Work out the finished part from the listing and answer in its coordinate system (mm). A direction names the side the tool comes from. Give positions to 0.01 mm unless a question says otherwise; leave off trailing zeros. Order: outer loops, then holes, each group sorted by start corner. A loop starts at its lowest first (then second) coordinate and runs counter-clockwise, first axis right, second up. Notation, with made-up numbers: (81.5, -37) - (138.5, -37) arc R22 cw to (138.5, -5) - close; hole circle Ø11 at (-15, 11). An arc over 180 degrees is marked (long way). Put each result on its own line as item: value.
```python
from build123d import *

# Parameters (mm, degrees)
SKETCH1_R           = 5
SKETCH1_R_2         = 6
SKETCH1_R_3         = 30
BOSS_EXTRUDE1_DEPTH = 6


with BuildPart() as part:
    # Sketch1 → Boss-Extrude1 (new body)
    with BuildSketch(Plane.XY):
        with BuildLine():
            Line((-183.863104209, -89.445070531), (-97.598804033, -2.338194347))
            ThreePointArc((-97.598804033, -2.338194347), (-66.500702639, 38.39419857), (-46.774466313, 85.692140845))
            Line((-46.774466313, 85.692140845), (-14.469848781, 203.952654329))
            ThreePointArc((-14.469848781, 203.952654329), (0, 215), (14.469848781, 203.952654329))
            Line((14.469848781, 203.952654329), (46.774466313, 85.692140845))
            ThreePointArc((46.774466313, 85.692140845), (66.500702639, 38.39419857), (97.598804033, -2.338194347))
            Line((97.598804033, -2.338194347), (183.863104209, -89.445070531))
            ThreePointArc((183.863104209, -89.445070531), (186.195461814, -107.5), (169.393255428, -114.507583798))
            Line((169.393255428, -114.507583798), (50.82433772, -83.353946498))
            ThreePointArc((50.82433772, -83.353946498), (0, -76.78839714), (-50.82433772, -83.353946498))
            Line((-50.82433772, -83.353946498), (-169.393255428, -114.507583798))
            ThreePointArc((-169.393255428, -114.507583798), (-186.195461814, -107.5), (-183.863104209, -89.445070531))
        make_face()
        with Locations((0, 200)):
            Circle(SKETCH1_R, mode=Mode.SUBTRACT)
        with Locations((173.205080757, -100)):
            Circle(SKETCH1_R, mode=Mode.SUBTRACT)
        with Locations((-173.205080757, -100)):
            Circle(SKETCH1_R, mode=Mode.SUBTRACT)
        with Locations((-35.355339059, 35.355339059)):
            Circle(SKETCH1_R_2, mode=Mode.SUBTRACT)
        with Locations((35.355339059, 35.355339059)):
            Circle(SKETCH1_R_2, mode=Mode.SUBTRACT)
        with Locations((35.355339059, -35.355339059)):
            Circle(SKETCH1_R_2, mode=Mode.SUBTRACT)
        with Locations((-35.355339059, -35.355339059)):
            Circle(SKETCH1_R_2, mode=Mode.SUBTRACT)
        Circle(SKETCH1_R_3, mode=Mode.SUBTRACT)
    extrude(amount=BOSS_EXTRUDE1_DEPTH)


solid = part.part
```
(1) Section B-B, the plane y = -100 is taken. Write down the section's boundary in (x, z).
Geometry check:
outline: (-188.21, 0) - (-178.21, 0) - (-178.21, 6) - (-188.21, 6) - close; (-168.21, 0) - (-114.18, 0) - (-114.18, 6) - (-168.21, 6) - close; (114.18, 0) - (168.21, 0) - (168.21, 6) - (114.18, 6) - close; (178.21, 0) - (188.21, 0) - (188.21, 6) - (178.21, 6) - close
(2) Straight lines are drawn through the part: line 1 (Y direction, x = -1, z = 3.2); line 2 (X direction, y = 8, z = 2.8); line 3 (Y direction, x = -129, z = 1.65). For each, find the intervals that lie inside material, in ascending order.
Geometry check:
line 1: y = -76.79 to -29.98, 29.98 to 195.1, 204.9 to 214.97
line 2: x = -88.06 to -28.91, 28.91 to 88.06
line 3: y = -103.89 to -34.05
(3) Section C-C, the plane z = 1.6 is taken. Count the separate pieces of the cut face and the enclosed holes in it, then the cut area to 3 significant figures.
Geometry check:
separate pieces: 1
enclosed holes: 8
area: 42,300 mm²
(4) A tool of negligible diameter and unlimited length cuts with its end or side. For faces 1 (the face through (110.94, -99.15, 2.96)), 2 (the face through (66.14, 39.02, 2.96)), from which of +Z, -Z, +X, -X, +Y, -Y can it reach the whole face along a straight path? Write none if from no direction.
Geometry check:
face 1: +Z, -Z, -Y
face 2: +Z, -Z, +X, +Y
(5) Section D-D, the plane y = -19 is taken. Write down the section's boundary in (x, z).
Geometry check:
outline: (-114.1, 0) - (-23.22, 0) - (-23.22, 6) - (-114.1, 6) - close; (23.22, 0) - (114.1, 0) - (114.1, 6) - (23.22, 6) - close
(6) Section A-A, the plane x = 0 is taken. Write down the section's boundary in (y, z), then the cut area to 3 significant figures.
Geometry check:
outline: (-76.79, 0) - (-30, 0) - (-30, 6) - (-76.79, 6) - close; (30, 0) - (195, 0) - (195, 6) - (30, 6) - close; (205, 0) - (215, 0) - (215, 6) - (205, 6) - close
area: 1,330 mm²
(7) Given pin 1 (13 mm diameter, centred on x = 173.21, y = -100, fed in from -Z); pin 2 (8 mm diameter, centred on x = 0, y = 200, fed in from -Z); pin 3 (1 mm diameter, centred on y = -23, z = 1, fed in from -X); pin 4 (1 mm diameter, centred on y = 100.5, z = 5, fed in from +X), each flat-ended and moving along its own axis, determine where each tip first touches the part or whether it passes through.
Geometry check:
pin 1: stops at z = 0
pin 2: passes through
pin 3: stops at x = -118.56
pin 4: stops at x = 42.87
(8) Determine the mould class of faces 3 (the face through (-109.279, -98.713, 2.958)), 4 (the face through (1, -35, 0)), 5 (the face through (34.05, -41.21, 2.96)), 6 (the face through (30.396, 145.65, 2.958)) for opening direction Y: pulls with the +Y half, pulls with the -Y half, needs draft (parallel to the pull), parting line crosses it, or undercut.
Geometry check:
face 3: pulls with the -Y half
face 4: needs draft
face 5: undercut
face 6: pulls with the +Y half
